The model under review builds one solid part; all positions refer to its coordinate system, in mm. Face numbers are marked on the shaded views. A direction names the side the tool comes from. Coordinates: 2 decimals unless noted, no trailing zeros. Loops run counter-clockwise (first coordinate to the right, second up) from the corner with the lowest first, then second, coordinate; pieces in that order, holes last. Notation, with made-up numbers: (85, 52) - (108, 52) arc R14 cw to (108, 74) - close; hole circle Ø9 at (68, 4.5). An arc over 180 degrees is marked (long way). Use a Markdown table: item, result. Add a question column.
1) To check wall thickness, follow L1, parallel to X at y = 1.5, z = 12; L2, parallel to X at y = 7.5, z = 13; L3, parallel to Y at x = 7, z = 1.5. State the ranges of each line that lie inside material, in increasing order. Write a range as [from, to].
2) Add section C-C, the plane z = 17.25. Give the boundary of the cut face in (x, y), and give its area (3 significant figures).
3) Add section D-D, the plane y = 16. Give the boundary of the cut face in (x, z), and give its area (3 significant figures).
4) Add section B-B, the plane x = 16. Give the boundary of the cut face in (y, z), and give its area (3 significant figures).
5) Clearance check with flat-ended pins moving along their axes: pin 1 (6.5 mm diameter, centred on y = 17, z = 13, fed in from -X); pin 2 (6.5 mm diameter, centred on y = 21, z = 10.5, fed in from +X); pin 3 (3 mm diameter, centred on y = 4.5, z = 2.5, fed in from -X). State where each tip first meets the part, or that it passes through.
6) Add section A-A, the plane z = 7.75. Give the boundary of the cut face in (x, y), and give its area (3 significant figures).
7) For the marked faces 1, 2 and 3, list the 3-axis set-ups (+Z, -Z, +X, -X, +Y, -Y) from which the entire face can be reached by the end or side of a thin tool; tool diameter is ignored.
8) The part is to be moulded in two halves that separate along Z. For the marked faces 4, 5 and 6, say which applies: pulls with the +Z half, pulls with the -Z half, needs draft (parallel to the pull), parting line crosses it, or undercut.
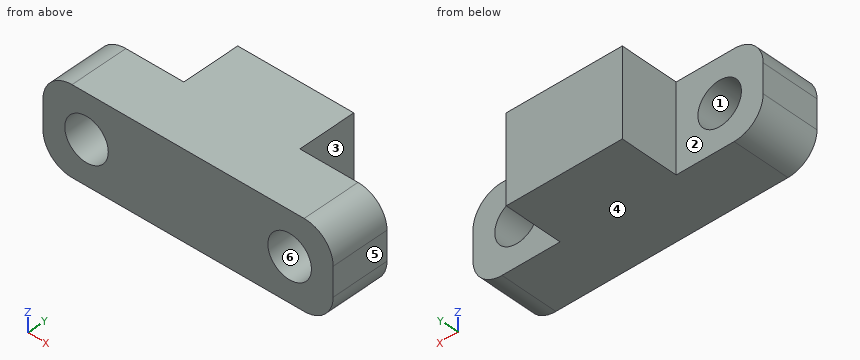
Autodesk Inventor part; units mm, degrees
ref_plane "YZ Plane" through (0, 0, 0) normal (1, 0, 0) x (0, 1, 0)
ref_plane "XZ Plane" through (0, 0, 0) normal (0, 1, 0) x (-1, 0, 0)
ref_plane "XY Plane" through (0, 0, 0) normal (0, 0, 1) x (1, 0, 0)
sketch "Sketch1" plane through (0, 0, 0) normal (0, 0, 1) x (1, 0, 0)
  line L0 (0, 0) -> (19.05, 0)
  line L1 (19.05, 12.7) -> (0, 12.7)
  line L2 (0, 12.7) -> (0, 0)
  line L3 (19.05, 0) -> (31.75, 0)
  line L4 (31.75, 0) -> (31.75, 25.4)
  line L5 (31.75, 25.4) -> (19.05, 25.4)
  line L6 (19.05, 25.4) -> (19.05, 12.7)
  dimension "d0" = 19.05
  dimension "d2" = 12.7
  dimension "d3" = 25.4
  dimension "d4" = 12.7
extrude "Extrusion1" add sketch "Sketch1" along normal blind 19.05
fillet "Fillet1" radius 6.35 2 edges at (0, 6.35, 19.05) (0, 6.35, 0)
sketch "Sketch2" plane through (19.05, 12.7, 19.05) normal (0, 1, 0) x (1, 0, 0)
  line L0 (0, 19.05) -> (-12.7, 19.05)
  line L1 (0, 19.05) -> (0, 0)
  circle A0 centre (-9.525, 9.525) radius 4.7625
  line L2 (0, 19.05) -> (-6.1574, 12.8926)
  line L3 (-12.8926, 6.1574) -> (-19.05, 0)
  line L4 (0, 0) -> (-6.1574, 6.1574)
  line L5 (-12.8926, 12.8926) -> (-19.05, 19.05)
  dimension "d8" = 9.525
extrude "Extrusion2" cut sketch "Sketch2" against normal through all contours A0
mirror "Mirror1" about plane through (31.75, 0, 0) normal (1, 0, 0) of "Extrusion1", "Extrusion2", "Fillet1"
properties part number "Mirror Feature Practice"
From the geometry:
| question | item | result |
|---|---|---|
| 1 | L1 | x = [0, 5.46], [13.59, 49.91], [58.04, 63.5] |
| 1 | L2 | x = [0.01, 6.27], [12.78, 50.72], [57.23, 63.49] |
| 1 | L3 | y = [0, 12.7] |
| 2 | outline | (1.92, 0) - (61.58, 0) - (61.58, 12.7) - (44.45, 12.7) - (44.45, 25.4) - (19.05, 25.4) - (19.05, 12.7) - (1.92, 12.7) - close |
| 2 | area | 1,080 mm^2 |
| 3 | outline | (19.05, 0) - (44.45, 0) - (44.45, 19.05) - (19.05, 19.05) - close |
| 3 | area | 484 mm^2 |
| 4 | outline | (0, 0) - (12.7, 0) - (12.7, 19.05) - (0, 19.05) - close |
| 4 | area | 242 mm^2 |
| 5 | pin 1 | stops at x = 19.05 |
| 5 | pin 2 | stops at x = 44.45 |
| 5 | pin 3 | stops at x = 0.45 |
| 6 | outline | (0, 0) - (5.11, 0) - (5.11, 12.7) - (0, 12.7) - close; (13.94, 0) - (49.56, 0) - (49.56, 12.7) - (44.45, 12.7) - (44.45, 25.4) - (19.05, 25.4) - (19.05, 12.7) - (13.94, 12.7) - close; (58.39, 0) - (63.5, 0) - (63.5, 12.7) - (58.39, 12.7) - close |
| 6 | area | 905 mm^2 |
| 7 | face 1 | +Y, -Y |
| 7 | face 2 | +Z, -Z, -X, +Y |
| 7 | face 3 | +Z, -Z, +X, +Y |
| 8 | face 4 | pulls with the -Z half |
| 8 | face 5 | needs draft |
| 8 | face 6 | undercut |
